Part model, mm, in its own coordinate system. A direction names the side the tool comes from. Coordinates: 2 decimals unless noted, no trailing zeros. Loops run counter-clockwise (first coordinate to the right, second up) from the corner with the lowest first, then second, coordinate; pieces in that order, holes last. Notation, with made-up numbers: (-12, 4.5) -> (3, 4.5) arc R19 cw to (3, 8.5) -> close; hole circle Ø3 at (-12, 8). An arc over 180 degrees is marked (long way). One line per item, written item: value. Start each with the question number.
from build123d import *

# Parameters (mm, degrees)
F0_W     = 12.7
F0_H     = 25.4
F2_DEPTH = 25.4
F1_W     = 25.4
F1_H     = 25.4
F3_DEPTH = 6.35
F4_R     = 5.08


with BuildPart() as f2:
    # F0 (on Top) → F2 (new body)
    with BuildSketch(Plane.XY):
        with Locations((6.35, 12.7)):
            Rectangle(F0_W, F0_H)
    extrude(amount=F2_DEPTH)

    # F1 (on Top) → F3 (join)
    with BuildSketch(Plane.XY):
        with Locations((25.376793, 12.7)):
            Rectangle(F1_W, F1_H)
    extrude(amount=F3_DEPTH)

    # F4
    f4_edges = [f2.edges().sort_by_distance(p)[0] for p in [
        (6.35, 0, 25.4),
        (6.35, 25.4, 25.4),
    ]]
    fillet(f4_edges, radius=F4_R)


solid = f2.part
1) Slice it at D-D (x = 15.5). Give the cut face in (y, z).
2) Slice it at C-C (z = 8.25). Give the cut face in (x, y).
3) Probe line 1 (Z direction, x = 13.5, y = 6.75); line 2 (X direction, y = 15.75, z = 7.5); line 3 (Y direction, x = 9, z = 21.25). List the from-to ranges inside material, lowest first. Write a range as from..to.
4) Slice it at A-A (x = 11.5). Give the cut face in (y, z).
5) Pin check, flat tip, straight feed: pin 1 Ø12.5 at (x, y) = (31.5, 15.5) entering from +Z. Stop position of the tip, or through.
6) Slice it at B-B (y = 9). Give the cut face in (x, z), then the cut area to 3 significant figures.
7) Tool access for faces 1 (the flat face through (12.7, 13, 16)), 2 (the cylindrical face through (6.439, 23.951, 23.872)): list every direction of +Z, -Z, +X, -X, +Y, -Y with a clear straight run to the whole face (end or side of a thin tool).
Check sheet entries:
1. outline: (0, 0) -> (25.4, 0) -> (25.4, 6.35) -> (0, 6.35) -> close
2. outline: (0, 0) -> (12.7, 0) -> (12.7, 25.4) -> (0, 25.4) -> close
3. line 1: z = 0..6.35
3. line 2: x = 0..12.7
3. line 3: y = 0.09..25.31
4. outline: (0, 0) -> (25.4, 0) -> (25.4, 20.32) arc R5.08 ccw to (20.32, 25.4) -> (5.08, 25.4) arc R5.08 ccw to (0, 20.32) -> close
5. pin 1: stops at z = 6.35
6. outline: (0, 0) -> (38.08, 0) -> (38.08, 6.35) -> (12.7, 6.35) -> (12.7, 25.4) -> (0, 25.4) -> close
6. area: 484 mm^2
7. face 1: +Z, +X, +Y, -Y
7. face 2: +Z, +X, -X, +Y
